from build123d import *

# Parameters (mm, degrees)
F3_DEPTH = 127
F5_DEPTH = 50.8


with BuildPart() as f1:
    # F0 (on Front) → F1 (revolve)
    with BuildSketch(Plane.XZ):
        with BuildLine():
            Line((0, 50.2139851451), (0, 0))
            Line((0, 0), (26.6106016934, 0))
            ThreePointArc((26.6106016934, 0), (47.0614731312, 20.4508714378), (26.6106016934, 40.9017428756))
            add(Edge.make_bspline(
                [(26.6106016934, 40.9017428756), (25.0362083316, 43.3508008718), (4.0366263129, 40.3783917427), (2.4622329511, 42.827449739)],
                knots=[0, 0, 0, 0, 24.2250296148, 24.2250296148, 24.2250296148, 24.2250296148], degree=3))
            add(Edge.make_bspline(
                [(2.4622329511, 42.827449739), (2.3834565669, 44.1874180439), (2.2387711309, 46.6852174669), (3.1683927039, 50.3577171038), (1.0311299141, 50.2607616454), (0, 50.2139851451)],
                knots=[0, 0, 0, 0, 0.3821769351, 0.7019290997, 1, 1, 1, 1], degree=3))
        make_face()
    revolve(axis=Axis((0, 0, 15.449039638), (0, 0, -1)))

    # F2 (on Right) → F3 (cut)
    with BuildSketch(Plane.YZ):
        Polygon((-19.8585987091, 33.3854667842), (-38.5659709573, 18.131762743), (-12.0878415182, 18.131762743), align=None)
        Polygon((25.6147161126, 33.3854667842), (13.814676553, 18.131762743), (34.2488847673, 18.131762743), align=None)
    extrude(amount=-F3_DEPTH, mode=Mode.SUBTRACT)

    # F4 (on Right) → F5 (cut)
    with BuildSketch(Plane.YZ):
        with BuildLine():
            add(Edge.make_bspline(
                [(29.3561853468, 13.2390642539), (32.4553857355, 10.7557147244), (20.3203773982, -0.772276878), (-12.8022721153, -1.9722855331), (-31.1402784868, 15.2170824896), (23.0618669435, 18.2826208766), (29.3561853468, 13.2390642539)],
                knots=[0, 0, 0, 0, 0.1761748956, 0.4813955957, 0.6421977451, 1, 1, 1, 1], degree=3))
        make_face()
    extrude(amount=-F5_DEPTH, mode=Mode.SUBTRACT)


solid = f1.part
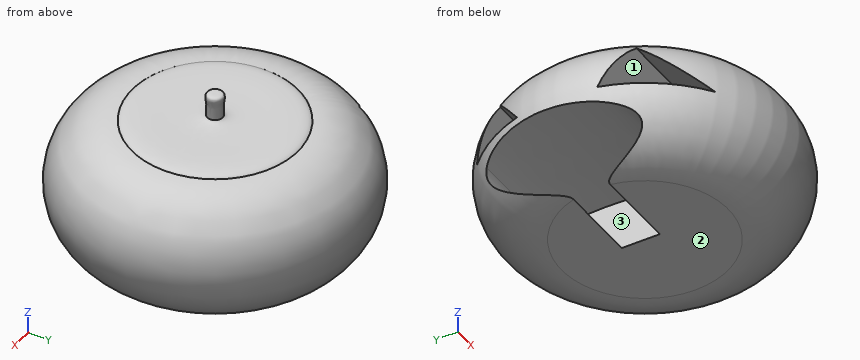
Verification items for the finished model (mm, model axes). Face numbers are marked on the shaded views. Give positions to 0.01 mm unless a question says otherwise; leave off trailing zeros. Write each loop counter-clockwise with the first axis right and the second up, starting at its lowest first coordinate (ties: lowest second). Pieces come first, ordered by that corner, then holes. Notation, with made-up numbers: (-2.5, -12) -> (41.5, -12) arc R20 ccw to (41.5, 13) -> close; hole circle Ø11 at (26.5, 40.5). An arc over 180 degrees is marked (long way). Use CSV: the item, a comma, the result in double quotes.
(1) Sectioned sample at B-B (x = -17). Give the number of separate pieces and of enclosed holes in the cut face, plus the area to 3 significant figures.
Derived:
separate pieces,"1"
enclosed holes,"2"
area,"2,230 mm^2"
(2) Go/stop test with flat-tipped pins: pin 1 (5 mm diameter, centred on y = 5.5, z = 9.5, fed in from -X); pin 2 (1.5 mm diameter, centred on x = -17, y = 3, fed in from -Z); pin 3 (8 mm diameter, centred on y = -32.5, z = 19.5, fed in from +X). Record where each tip stops, or that it passes through.
Derived:
pin 1,"stops at x = 0"
pin 2,"stops at z = 15.73"
pin 3,"stops at x = 37.43"
(3) Release check for a two-part mould opening along Y. For the marked faces 1, 2 and 3 record: +Y half, -Y half, draft (parallel to the pull), parting line (faces both ways), or undercut.
Derived:
face 1,"undercut"
face 2,"draft"
face 3,"undercut"
(4) Sectioned sample at A-A (z = 26.5). Record the cut outline in (x, y), plus the area to 3 significant figures.
Derived:
outline,"(-43.15, -16.35) -> (0, -16.35) -> (0, -28.3) -> (-36.45, -28.3) arc R46.15 ccw (long way) to (-35.48, 29.51) -> (0, 29.51) -> (0, 20.29) -> (-41.45, 20.29) arc R46.15 ccw to start"
area,"5,850 mm^2"
(5) Material ranges on L1, parallel to Z at x = -11, y = 26; L2, parallel to Y at x = -31, z = 20; L3, parallel to Z at x = -20, y = -31, recorded low to high.
Derived:
L1,"z = 0.06 to 6.01, 14.71 to 18.13, 32.7 to 40.84"
L2,"y = -13.04 to 15.26, 33.19 to 35.4"
L3,"z = 2.77 to 18.13, 24.3 to 38.13"
